Input: part model. Units: mm. Frame: model coordinates. Coordinates: 2 decimals unless noted, no trailing zeros. Order: outer loops, then holes, each group sorted by start corner. A loop starts at its lowest first (then second) coordinate and runs counter-clockwise, first axis right, second up. Notation, with made-up numbers: (59, 70.5) - (79, 70.5) arc R16 cw to (79, 96.5) - close; hole circle Ø10 at (1, -33). An arc over 180 degrees is marked (long way). Use a Markdown table: item, result. Add a question column.
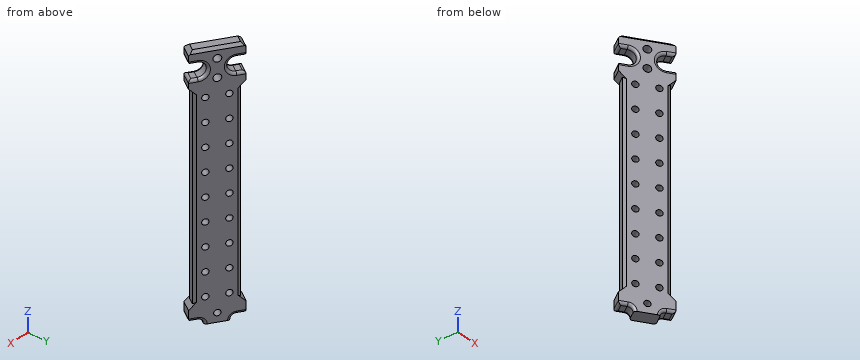
from build123d import *

# Parameters (mm, degrees)
BOSS_EXTRU_1_OUTLINE_R   = 2.75
BOSS_EXTRU_1_OUTLINE_R_2 = 2.3
BOSS_EXTRU_1_DEPTH       = 10
ESQUISSE2_R              = 2.3
ENL_V_MAT_EXTRU_1_DEPTH  = 191.138157298
CONG_1_R                 = 2
CHANFREIN1_SIZE          = 2
CONG_2_R                 = 2


# Read off the part's stored shape, not the designer's step: Boss.-Extru.1
with BuildPart() as part:
    # Boss.-Extru.1 outline → Boss.-Extru.1 (new body)
    with BuildSketch(Plane(origin=(0.807648755, 1.292238009, 0), x_dir=(0.8479983040028684, -0.5299989400067315, 0), z_dir=(0.5299989400067315, 0.8479983040028684, 0))):
        with BuildLine():
            Line((-3.319738136, 181.25), (-9.244866887, 181.25))
            ThreePointArc((-9.244866887, 181.25), (-11.896517316, 182.348349571), (-12.994866887, 185))
            Line((-12.994866887, 185), (-29.644053825, 185))
            ThreePointArc((-29.644053825, 185), (-30.742403396, 182.348349571), (-33.394053825, 181.25))
            Line((-33.394053825, 181.25), (-39.319182576, 181.25))
            Line((-39.319182576, 181.25), (-39.319182576, 173))
            Line((-39.319182576, 173), (-36.319182576, 170))
            Line((-36.319182576, 170), (-36.319182576, 15))
            Line((-36.319182576, 15), (-39.319182576, 12))
            Line((-39.319182576, 12), (-39.319182576, 5.75))
            Line((-39.319182576, 5.75), (-33.394053825, 5.75))
            ThreePointArc((-33.394053825, 5.75), (-27.644053825, 0), (-33.394053825, -5.75))
            Line((-33.394053825, -5.75), (-39.319182576, -5.75))
            Line((-39.319182576, -5.75), (-39.319182576, -12))
            Line((-39.319182576, -12), (-36.319182576, -15))
            Line((-36.319182576, -15), (-6.319738136, -15))
            Line((-6.319738136, -15), (-3.319738136, -12))
            Line((-3.319738136, -12), (-3.319738136, -5.75))
            Line((-3.319738136, -5.75), (-9.244866887, -5.75))
            ThreePointArc((-9.244866887, -5.75), (-14.994866887, 0), (-9.244866887, 5.75))
            Line((-9.244866887, 5.75), (-3.319738136, 5.75))
            Line((-3.319738136, 5.75), (-3.319738136, 12))
            Line((-3.319738136, 12), (-6.319738136, 15))
            Line((-6.319738136, 15), (-6.319738136, 170))
            Line((-6.319738136, 170), (-3.319738136, 173))
            Line((-3.319738136, 173), (-3.319738136, 181.25))
        make_face()
        with Locations((-21.319460356, -7)):
            Circle(BOSS_EXTRU_1_OUTLINE_R, mode=Mode.SUBTRACT)
        with Locations((-21.319460356, 7)):
            Circle(BOSS_EXTRU_1_OUTLINE_R, mode=Mode.SUBTRACT)
        with Locations((-21.319460356, 178)):
            Circle(BOSS_EXTRU_1_OUTLINE_R_2, mode=Mode.SUBTRACT)
    extrude(amount=BOSS_EXTRU_1_DEPTH)

    # Esquisse2 → Enlèv. mat.-Extru.1 (cut, through all)
    with BuildSketch(Plane(origin=(6.107638155, 9.772221049, 0), x_dir=(0.8479983040028684, -0.5299989400067316, 0), z_dir=(0.5299989400067316, 0.8479983040028684, 0))):
        with Locations(Location((-28.819321466, 146.875, 0), (0, 0, 180))):
            Circle(ESQUISSE2_R)
        with Locations(Location((-13.819599246, 146.875, 0), (0, 0, 180))):
            Circle(ESQUISSE2_R)
        with Locations(Location((-28.819321466, 128.75, 0), (0, 0, 180))):
            Circle(ESQUISSE2_R)
        with Locations(Location((-13.819599246, 128.75, 0), (0, 0, 180))):
            Circle(ESQUISSE2_R)
        with Locations(Location((-28.819321466, 110.625, 0), (0, 0, 180))):
            Circle(ESQUISSE2_R)
        with Locations(Location((-13.819599246, 110.625, 0), (0, 0, 180))):
            Circle(ESQUISSE2_R)
        with Locations(Location((-28.819321466, 92.5, 0), (0, 0, 180))):
            Circle(ESQUISSE2_R)
        with Locations(Location((-13.819599246, 92.5, 0), (0, 0, 180))):
            Circle(ESQUISSE2_R)
        with Locations(Location((-28.819321466, 74.375, 0), (0, 0, 180))):
            Circle(ESQUISSE2_R)
        with Locations(Location((-13.819599246, 74.375, 0), (0, 0, 180))):
            Circle(ESQUISSE2_R)
        with Locations(Location((-13.819599246, 56.25, 0), (0, 0, 180))):
            Circle(ESQUISSE2_R)
        with Locations(Location((-13.819599246, 38.125, 0), (0, 0, 180))):
            Circle(ESQUISSE2_R)
        with Locations(Location((-13.819599246, 20, 0), (0, 0, 180))):
            Circle(ESQUISSE2_R)
        with Locations(Location((-28.819321466, 38.125, 0), (0, 0, 180))):
            Circle(ESQUISSE2_R)
        with Locations(Location((-28.819321466, 20, 0), (0, 0, 180))):
            Circle(ESQUISSE2_R)
        with Locations(Location((-28.819321466, 56.25, 0), (0, 0, 180))):
            Circle(ESQUISSE2_R)
        with Locations(Location((-28.819321466, 165, 0), (0, 0, 180))):
            Circle(ESQUISSE2_R)
        with Locations(Location((-13.819599246, 165, 0), (0, 0, 180))):
            Circle(ESQUISSE2_R)
    extrude(amount=-ENL_V_MAT_EXTRU_1_DEPTH, mode=Mode.SUBTRACT)

    # Congé1
    cong_1_edges = [part.edges().sort_by_distance(p)[0] for p in [
        (-3.980588352, 16.077362616, -182.348349571),
        (0.78025628, 13.10183472, -181.25),
        (-19.961867785, 26.065662262, -182.348349571),
        (-24.722712418, 29.041190157, -181.25),
        (-4.51973312, 4.62185168, -181.25),
        (-30.022701818, 20.561207117, -181.25),
        (-25.261857185, 17.585679222, -182.348349571),
        (-9.280577752, 7.597379576, -182.348349571),
        (0.642511146, 7.291687222, -181.25),
        (-29.884956684, 26.371354616, -181.25),
    ]]
    fillet(cong_1_edges, radius=CONG_1_R)

    # Chanfrein1
    chanfrein1_edges = [part.edges().sort_by_distance(p)[0] for p in [
        (0.748510934, 13.121675562, -92.5),
        (-4.551478466, 4.641692522, -92.5),
        (-17.271217469, 12.591529399, 15),
        (-29.990956472, 20.541366276, -92.5),
        (-24.690967072, 29.021349316, -92.5),
        (-11.971228069, 21.071512439, 15),
    ]]
    chamfer(chanfrein1_edges, length=CHANFREIN1_SIZE)

    # Congé2
    cong_2_edges = [part.edges().sort_by_distance(p)[0] for p in [
        (0.78025628, 13.10183472, 5.75),
        (-6.607983534, 17.719484604, 0),
        (0.78025628, 13.10183472, -5.75),
        (-4.51973312, 4.62185168, -5.75),
        (-11.907972934, 9.239501564, 0),
        (-4.51973312, 4.62185168, 5.75),
        (-30.022701818, 20.561207117, 5.75),
        (-22.634462004, 15.943557233, 0),
        (-30.022701818, 20.561207117, -5.75),
        (0.642511146, 7.291687222, -5.75),
        (0.642511146, 7.291687222, 5.75),
        (-29.884956684, 26.371354616, 5.75),
        (-29.884956684, 26.371354616, -5.75),
        (-24.722712418, 29.041190157, -5.75),
        (-17.334472604, 24.423540273, 0),
        (-24.722712418, 29.041190157, 5.75),
    ]]
    fillet(cong_2_edges, radius=CONG_2_R)


solid = part.part
1) Material intervals for L1, parallel to Z at x = -1.5, y = 11.25; L2, parallel to X at y = 23.5, z = -166.5; L3, parallel to Y at x = -23, z = -146, sorted ascending.
2) Contact query for flat-ended pins moving along their axis: P1, Ø5, axis at x = -5.5, z = -59, coming from the +Y side; P2, Ø5, axis at x = -25, y = 23, coming from the -Z side; P3, Ø7, axis at x = -3, y = 9, coming from the -Z side. Output: stop coordinate, or through.
3) Cut plane A-A (z = -83). Return the cut outline in (x, y), and give its area (3 significant figures).
Computed:
| question | item | result |
|---|---|---|
| 1 | L1 | z = -181.25 to -5.75, 5.75 to 15 |
| 1 | L2 | x = -28.14 to -21.35, -17.24 to -15.86 |
| 1 | L3 | y = 21.59 to 27.96 |
| 2 | P1 | stops at y = 18.59 |
| 2 | P2 | stops at z = -182.21 |
| 2 | P3 | stops at z = -181.59 |
| 3 | outline | (-28.93, 22.24) - (-28.29, 19.48) - (-6.25, 5.7) - (-3.49, 6.34) - (-0.31, 11.43) - (-0.95, 14.18) - (-22.99, 27.96) - (-25.75, 27.33) - close |
| 3 | area | 292 mm2 |
